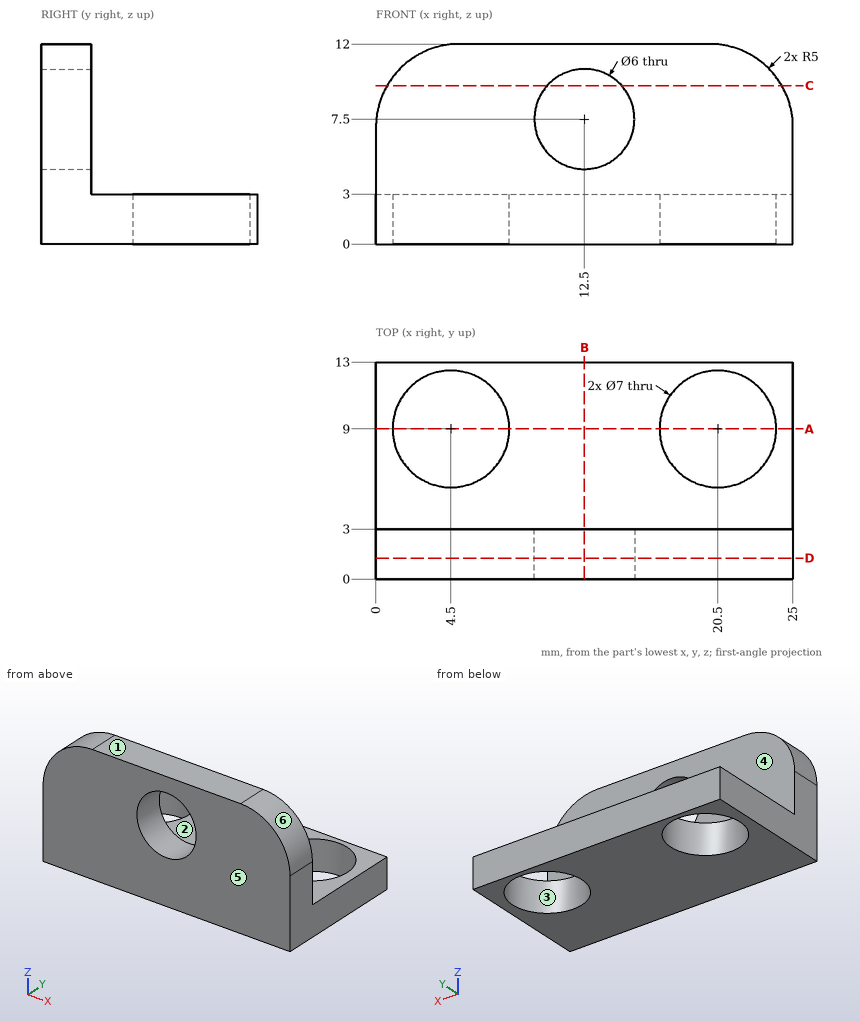
The drawing under review shows one solid part. Ordinate dimensions are in mm from its lowest x, y, z. A direction names the side the tool comes from. Round coordinates to 2 decimals unless told otherwise and drop trailing zeros. Order: outer loops, then holes, each group sorted by start corner. A loop starts at its lowest first (then second) coordinate and runs counter-clockwise, first axis right, second up. Notation, with made-up numbers: (-13, 9) -> (26, 9) arc R7 cw to (26, 17) -> close; hole circle Ø8 at (-13, 52.25). An arc over 180 degrees is marked (long way). Use a Markdown table: item, result.
Q1. We need section A-A on y = 9. Write out the cut boundary in (x, z).
Values:
| item | result |
|---|---|
| outline | (0, 0) -> (1, 0) -> (1, 3) -> (0, 3) -> close; (8, 0) -> (17, 0) -> (17, 3) -> (8, 3) -> close; (24, 0) -> (25, 0) -> (25, 3) -> (24, 3) -> close |
Q2. Tool access review of the marked faces 1 and 2: name each direction out of +Z, -Z, +X, -X, +Y, -Y from which nothing blocks a thin tool from reaching the whole face with its end or side.
Values:
| item | result |
|---|---|
| face 1 | +Z, +X, -X, +Y, -Y |
| face 2 | +Z, +X, -X, +Y |
Q3. Mouldability with a two-part tool opening along Y and no side actions: class the marked faces 3, 4, 5 and 6 as +Y half, -Y half, draft (parallel to the pull), parting line (faces both ways), or undercut.
Values:
| item | result |
|---|---|
| face 3 | undercut |
| face 4 | +Y half |
| face 5 | -Y half |
| face 6 | draft |
Q4. We need section C-C on z = 9.5. Write out the cut boundary in (x, y).
Values:
| item | result |
|---|---|
| outline | (0.67, 0) -> (10.26, 0) -> (10.26, 3) -> (0.67, 3) -> close; (14.74, 0) -> (24.33, 0) -> (24.33, 3) -> (14.74, 3) -> close |
Q5. Clearance check with a flat-ended pin moving along its axis: P1, Ø4.5, axis at x = 15, z = 9.5, coming from the +Y side. State where the tip first meets the part, or that it passes through.
Values:
| item | result |
|---|---|
| P1 | stops at y = 3 |
Q6. For line 1 (Y direction, x = 20.5, z = 1.15); line 2 (Y direction, x = 5.25, z = 7.5), list the stretches that pass through material, from the lowest coordinate up.
Values:
| item | result |
|---|---|
| line 1 | y = 0 to 5.5, 12.5 to 13 |
| line 2 | y = 0 to 3 |
Q7. We need section B-B on x = 12.5. Write out the cut boundary in (y, z).
Values:
| item | result |
|---|---|
| outline | (0, 0) -> (13, 0) -> (13, 3) -> (3, 3) -> (3, 4.5) -> (0, 4.5) -> close; (0, 10.5) -> (3, 10.5) -> (3, 12) -> (0, 12) -> close |
Q8. We need section D-D on y = 1.25. Write out the cut boundary in (x, z).
Values:
| item | result |
|---|---|
| outline | (0, 0) -> (25, 0) -> (25, 7) arc R5 ccw to (20, 12) -> (5, 12) arc R5 ccw to (0, 7) -> close; hole circle Ø6 at (12.5, 7.5) |
